Here's how the part is built. I have some questions about the finished solid (model axes, mm). A direction names the side the tool comes from. Round coordinates to 2 decimals unless told otherwise and drop trailing zeros. Order: outer loops, then holes, each group sorted by start corner. A loop starts at its lowest first (then second) coordinate and runs counter-clockwise, first axis right, second up.
```python
from build123d import *

# Parameters (mm, degrees)
SKETCH001_R  = 6.35
PAD_DEPTH    = 7.62
SKETCH_R     = 7.9375
PAD001_DEPTH = 15.24
CHAMFER_SIZE = 1.27


with BuildPart() as part:
    # Sketch001 → Pad (new body)
    with BuildSketch(Plane.XY):
        Circle(SKETCH001_R)
    extrude(amount=PAD_DEPTH)

    # Sketch → Pad001 (join)
    with BuildSketch(Plane.XY):
        Circle(SKETCH_R)
    extrude(amount=-PAD001_DEPTH)

    # Chamfer
    chamfer_edges = [part.edges().sort_by_distance(p)[0] for p in [
        (-6.35, 0, 7.62),
    ]]
    chamfer(chamfer_edges, length=CHAMFER_SIZE)


solid = part.part
```
1) I need wall thicknesses on line 1 (Z direction, x = 5.75, y = -5); line 2 (X direction, y = -0.25, z = 6.25); line 3 (X direction, y = 3.25, z = -3.5). Which ranges of each line are inside material? Lowest first, please.
2) If we section it at D-D (z = 5.5): Write out the boundary of the cut face in (x, y).
3) If we section it at A-A (x = 0): Write out the boundary of the cut face in (y, z), plus the area to 3 significant figures.
4) I'm going to push flat-ended pins straight in: pin 1 (6 mm diameter, centred on x = -4.5, z = 0.5, fed in from -Y); pin 2 (2 mm diameter, centred on y = 1.5, z = 5.5, fed in from +X); pin 3 (6 mm diameter, centred on x = -6.5, z = -9, fed in from -Y). Where does each tip first touch, or does it pass through?
5) If we section it at C-C (z = -6.5): Write out the boundary of the cut face in (x, y) (1 decimal), plus the area to 3 significant figures.
6) For faces 1 (the flat face through (0, 0, -15.24)), 2 (the cylindrical face through (-1.38, -6.2, 3.13)), which set-ups out of +Z, -Z, +X, -X, +Y, -Y let a thin tool reach every point of the face, with its end or its side?
Solutions:
1. line 1: z = -15.24 to 0
1. line 2: x = -6.35 to 6.35
1. line 3: x = -7.24 to 7.24
2. outline: circle Ø12.7 at (0, 0)
3. outline: (-7.94, -15.24) - (7.94, -15.24) - (7.94, 0) - (6.35, 0) - (6.35, 6.35) - (5.08, 7.62) - (-5.08, 7.62) - (-6.35, 6.35) - (-6.35, 0) - (-7.94, 0) - close
3. area: 337 mm2
4. pin 1: stops at y = -7.79
4. pin 2: stops at x = 6.33
4. pin 3: stops at y = -7.12
5. outline: circle Ø15.9 at (0, 0)
5. area: 198 mm2
6. face 1: -Z, +X, -X, +Y, -Y
6. face 2: +Z
